Check sheet for the modelled part. Datum: model origin and axes. Units: mm. A direction names the side the tool comes from. Round coordinates to 2 decimals unless told otherwise and drop trailing zeros. Write each loop counter-clockwise with the first axis right and the second up, starting at its lowest first coordinate (ties: lowest second). Pieces come first, ordered by that corner, then holes. Notation, with made-up numbers: M 13,-34 L 55,-34 A33 ccw 55,-1 Z; hole C 60.25,65 d5. An arc over 180 degrees is marked long. Answer in a Markdown table with one row per item.
Autodesk Inventor part; units mm, degrees
ref_plane "YZ Plane" through (0, 0, 0) normal (1, 0, 0) x (0, 1, 0)
ref_plane "XZ Plane" through (0, 0, 0) normal (0, 1, 0) x (-1, 0, 0)
ref_plane "XY Plane" through (0, 0, 0) normal (0, 0, 1) x (1, 0, 0)
sketch "スケッチ1" plane through (0, 0, 0) normal (0, 0, 1) x (1, 0, 0)
  circle A0 centre (0, 0) radius 1.5
  dimension "d0" = 3
extrude "押し出し1" add sketch "スケッチ1" along normal blind 6
sketch "スケッチ2" plane through (0, 0, 6) normal (0, 0, 1) x (1, 0, 0)
  circle A0 centre (0, 0) radius 1.5
  circle A1 centre (0, 0) radius 3
  dimension "d3" = 6
extrude "押し出し2" add sketch "スケッチ2" along normal blind 1.75 contours A0 | A1
thread "ねじ1"
chamfer "面取り1" distance 1.5 angle 45 1 edges at (-3, 0, 6)
sketch "スケッチ4" plane through (0, 0, 0) normal (0, 0, -1) x (-1, 0, 0)
  circle A0 centre (0, 0) radius 1.5
extrude "押し出し4" cut sketch "スケッチ4" against normal blind 2
sketch "スケッチ5" plane through (0, 0, 2) normal (0, 0, -1) x (-1, 0, 0)
  circle A0 centre (0, 0) radius 1.5
extrude "押し出し5" cut sketch "スケッチ5" against normal blind 1.75
properties part number "SB　4mm皿ネジ(高い)" material "Steel, Mild"
1. Section check C-C, the plane z = 5.05. Record the cut outline in (x, y), and give its area (3 significant figures).
Found:
| item | result |
|---|---|
| outline | C 0,0 d3 |
| area | 7.07 mm2 |
2. Scan lines: L1, parallel to Y at x = 0.3, z = 4.05; L2, parallel to Z at x = -0.6, y = 2.5; L3, parallel to X at y = -0.5, z = 6.6. Record each from-to range of solid material in increasing order.
Found:
| item | result |
|---|---|
| L1 | y = -1.47 to 1.47 |
| L2 | z = 7.07 to 7.75 |
| L3 | x = -2.04 to 2.04 |
3. Section check D-D, the plane z = 6.25. Record the cut outline in (x, y).
Found:
| item | result |
|---|---|
| outline | C 0,0 d3.5 |
4. Go/stop test with a flat-tipped pin: pin 1 (1.5 mm diameter, centred on x = -1.5, z = 4.5, fed in from +Y). Record where the tip stops, or that it passes through.
Found:
| item | result |
|---|---|
| pin 1 | stops at y = 1.3 |
5. Access from +Z, -Z, +X, -X, +Y, -Y to the whole of each face (thin tool, end or side, straight path). Record for faces 1 (the face through (0, 0, 3.75)), 2 (the face through (-1.5, -0.07, 4.86)).
Found:
| item | result |
|---|---|
| face 1 | -Z, +X, -X, +Y, -Y |
| face 2 | -Z |
